```python
from build123d import *

# Parameters (mm, degrees)
F0_R     = 65
F1_DEPTH = 240
F0_R_2   = 1.25
F2_DEPTH = 2.5
F3_D     = 5


with BuildPart() as f1:
    # F0 (on Top) → F1 (new body)
    with BuildSketch(Plane.XY):
        with BuildLine():
            ThreePointArc((70, 0), (49.497475, 49.497475), (0, 70))
            ThreePointArc((0, 70), (-49.497475, 49.497475), (-70, 0))
            ThreePointArc((-70, 0), (-49.497475, -49.497475), (0, -70))
            ThreePointArc((0, -70), (49.497475, -49.497475), (70, 0))
        make_face()
        Circle(F0_R, mode=Mode.SUBTRACT)
    extrude(amount=F1_DEPTH)

    # F0 (on Top) → F2 (join)
    with BuildSketch(Plane.XY):
        Circle(F0_R)
        Circle(F0_R_2, mode=Mode.SUBTRACT)
    extrude(amount=F2_DEPTH)

    # F3 (through all)
    with Locations(Plane(origin=(0, 0, 0), x_dir=(1, 0, 0), z_dir=(0, 0, -1))):
        with Locations((0, 0)):
            Hole(F3_D / 2)


solid = f1.part
```
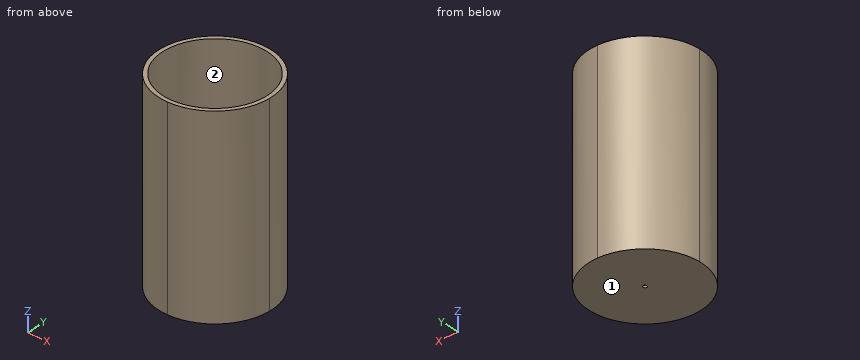
Design review of the part built by this model. Coordinates are the model's own, in mm. Face numbers are marked on the shaded views. Give positions to 0.01 mm unless a question says otherwise; leave off trailing zeros. Loops run counter-clockwise (first coordinate to the right, second up) from the corner with the lowest first, then second, coordinate; pieces in that order, holes last. Notation, with made-up numbers: (11, -32) -> (24, -32) arc R29 cw to (24, -12) -> close; hole circle Ø7 at (67.5, 21). An arc over 180 degrees is marked (long way). One line per item, written item: value.
Q1. Draft analysis for pull direction Y (two halves, no side actions). For the marked faces 1 and 2, state which applies: pulls with the +Y half, pulls with the -Y half, needs draft (parallel to the pull), parting line crosses it, or undercut.
Numbers:
face 1: needs draft
face 2: undercut
Q2. We need section B-B on y = 52. Give the boundary of the cut face in (x, z).
Numbers:
outline: (-46.86, 0) -> (46.86, 0) -> (46.86, 240) -> (39, 240) -> (39, 2.5) -> (-39, 2.5) -> (-39, 240) -> (-46.86, 240) -> close
Q3. For L1, parallel to X at y = 0.5, z = 155.5; L2, parallel to Z at x = -18, y = -19.5; L3, parallel to X at y = -47, z = 97, list the stretches that pass through material, from the lowest coordinate up.
Numbers:
L1: x = -70 to -65, 65 to 70
L2: z = 0 to 2.5
L3: x = -51.87 to -44.9, 44.9 to 51.87
Q4. We need section C-C on x = 34.5. Give the boundary of the cut face in (y, z), and give its area (3 significant figures).
Numbers:
outline: (-60.91, 0) -> (60.91, 0) -> (60.91, 240) -> (55.09, 240) -> (55.09, 2.5) -> (-55.09, 2.5) -> (-55.09, 240) -> (-60.91, 240) -> close
area: 3,070 mm^2
Q5. For pin 1 Ø5 at (y, z) = (41.5, 52) entering from +X; pin 2 Ø10 at (x, z) = (39.5, 165.5) entering from -Y; pin 3 Ø10 at (x, z) = (-16.5, 192) entering from +Y, all flat-tipped, find the tip position at first contact; note any pin that passes through.
Numbers:
pin 1: stops at x = 58.13
pin 2: stops at y = -60.91
pin 3: stops at y = 69.05
Q6. We need section A-A on z = 76. Give the boundary of the cut face in (x, y).
Numbers:
outline: (-70, 0) arc R70 ccw to (0, -70) arc R70 ccw to (70, 0) arc R70 ccw to (0, 70) arc R70 ccw to start; hole circle Ø130 at (0, 0)
